from build123d import *

# Parameters (mm, degrees)
F0_W      = 27
F0_H      = 15.9
F0_W_2    = 15.9
F0_H_2    = 27
F0_W_3    = 3
F0_H_3    = 3
F1_DEPTH  = 21.9
F2_DEPTH  = 51.8
F3_R      = 7.95
F6_DEPTH  = 30
F7_DEPTH  = 30
F4_R      = 7.9
F8_DEPTH  = 30
F10_DEPTH = 58.2
F11_W     = 3
F11_H     = 13.3
F13_R     = 1.5
F17_DEPTH = 51.9


with BuildPart() as f1:
    # F0 (on Front) → F1 (new body)
    with BuildSketch(Plane.XZ):
        with BuildLine():
            Line((-34.3576915575, 15.9), (-42.3076915575, 15.9))
            Line((-42.3076915575, 15.9), (-42.3076915575, 7.9499999931))
            ThreePointArc((-42.3076915575, 7.9499999931), (-39.9791904704, 13.571498908), (-34.3576915575, 15.9))
        make_face()
        with BuildLine():
            ThreePointArc((-34.3576915575, 15.9), (-39.9791904704, 13.571498908), (-42.3076915575, 7.9499999931))
            ThreePointArc((-42.3076915575, 7.9499999931), (-39.9791904655, 2.3285010871), (-34.3576915575, 0))
            ThreePointArc((-34.3576915575, 0), (-28.7361926471, 2.3285010896), (-26.4076915575, 7.95))
            ThreePointArc((-26.4076915575, 7.95), (-28.7361926471, 13.5714989104), (-34.3576915575, 15.9))
        make_face()
        Polygon((-42.3076915575, 18.9), (-42.3076915575, 45.9), (-26.4076915575, 45.9), (-26.4076915575, 18.9), (-23.4076915575, 18.9), (-23.4076915575, 48.9), (-45.3076915575, 48.9), (-45.3076915575, 18.9), align=None)
        with Locations((-9.9076915575, 7.95)):
            Rectangle(F0_W, F0_H)
        with Locations((-34.3576915575, 32.4)):
            Rectangle(F0_W_2, F0_H_2)
        with BuildLine():
            ThreePointArc((-34.3576915575, 0), (-39.9791904655, 2.3285010871), (-42.3076915575, 7.9499999931))
            Line((-42.3076915575, 7.9499999931), (-42.3076915575, 0))
            Line((-42.3076915575, 0), (-34.3576915575, 0))
        make_face()
        with BuildLine():
            Line((-26.4076915575, 0), (-26.4076915575, 7.95))
            ThreePointArc((-26.4076915575, 7.95), (-28.7361926471, 2.3285010896), (-34.3576915575, 0))
            Line((-34.3576915575, 0), (-26.4076915575, 0))
        make_face()
        with BuildLine():
            Line((-26.4076915575, 7.95), (-26.4076915575, 15.9))
            Line((-26.4076915575, 15.9), (-34.3576915575, 15.9))
            ThreePointArc((-34.3576915575, 15.9), (-28.7361926471, 13.5714989104), (-26.4076915575, 7.95))
        make_face()
        Polygon((6.5923084425, 18.9), (-23.4076915575, 18.9), (-23.4076915575, 15.9), (3.5923084425, 15.9), (3.5923084425, 0), (-23.4076915575, 0), (-23.4076915575, -3), (6.5923084425, -3), align=None)
        Polygon((-26.4076915575, 18.9), (-42.3076915575, 18.9), (-42.3076915575, 15.9), (-34.3576915575, 15.9), (-26.4076915575, 15.9), align=None)
        Polygon((-23.4076915575, 15.9), (-26.4076915575, 15.9), (-26.4076915575, 7.95), (-26.4076915575, 0), (-23.4076915575, 0), align=None)
        Polygon((-42.3076915575, 15.9), (-42.3076915575, 18.9), (-45.3076915575, 18.9), (-45.3076915575, -3), (-23.4076915575, -3), (-23.4076915575, 0), (-26.4076915575, 0), (-34.3576915575, 0), (-42.3076915575, 0), (-42.3076915575, 7.9499999931), align=None)
        with Locations((-24.9076915575, 17.4)):
            Rectangle(F0_W_3, F0_H_3)
    extrude(amount=F1_DEPTH)

    # F0 (on Front) → F2 (join)
    with BuildSketch(Plane.XZ):
        Polygon((-42.3076915575, 15.9), (-42.3076915575, 18.9), (-45.3076915575, 18.9), (-45.3076915575, -3), (-23.4076915575, -3), (-23.4076915575, 0), (-26.4076915575, 0), (-34.3576915575, 0), (-42.3076915575, 0), (-42.3076915575, 7.9499999931), align=None)
        with BuildLine():
            ThreePointArc((-34.3576915575, 15.9), (-39.9791904704, 13.571498908), (-42.3076915575, 7.9499999931))
            ThreePointArc((-42.3076915575, 7.9499999931), (-39.9791904655, 2.3285010871), (-34.3576915575, 0))
            ThreePointArc((-34.3576915575, 0), (-28.7361926471, 2.3285010896), (-26.4076915575, 7.95))
            ThreePointArc((-26.4076915575, 7.95), (-28.7361926471, 13.5714989104), (-34.3576915575, 15.9))
        make_face()
        Polygon((-26.4076915575, 18.9), (-42.3076915575, 18.9), (-42.3076915575, 15.9), (-34.3576915575, 15.9), (-26.4076915575, 15.9), align=None)
        Polygon((-23.4076915575, 15.9), (-26.4076915575, 15.9), (-26.4076915575, 7.95), (-26.4076915575, 0), (-23.4076915575, 0), align=None)
        with Locations((-24.9076915575, 17.4)):
            Rectangle(F0_W_3, F0_H_3)
        with BuildLine():
            Line((-26.4076915575, 7.95), (-26.4076915575, 15.9))
            Line((-26.4076915575, 15.9), (-34.3576915575, 15.9))
            ThreePointArc((-34.3576915575, 15.9), (-28.7361926471, 13.5714989104), (-26.4076915575, 7.95))
        make_face()
        with BuildLine():
            Line((-34.3576915575, 15.9), (-42.3076915575, 15.9))
            Line((-42.3076915575, 15.9), (-42.3076915575, 7.9499999931))
            ThreePointArc((-42.3076915575, 7.9499999931), (-39.9791904704, 13.571498908), (-34.3576915575, 15.9))
        make_face()
        with BuildLine():
            ThreePointArc((-34.3576915575, 0), (-39.9791904655, 2.3285010871), (-42.3076915575, 7.9499999931))
            Line((-42.3076915575, 7.9499999931), (-42.3076915575, 0))
            Line((-42.3076915575, 0), (-34.3576915575, 0))
        make_face()
        with BuildLine():
            Line((-26.4076915575, 0), (-26.4076915575, 7.95))
            ThreePointArc((-26.4076915575, 7.95), (-28.7361926471, 2.3285010896), (-34.3576915575, 0))
            Line((-34.3576915575, 0), (-26.4076915575, 0))
        make_face()
    extrude(amount=F2_DEPTH)

    # F3 (on face) → F6 (cut)
    with BuildSketch(Plane.XZ.offset(51.8)):
        with Locations((-34.3576915575, 7.95)):
            Circle(F3_R)
    extrude(amount=-F6_DEPTH, mode=Mode.SUBTRACT)

    # F5 (on face) → F7 (cut)
    with BuildSketch(Plane.YZ.offset(6.5923084425)):
        with BuildLine():
            ThreePointArc((-3, 7.95), (-5.3285010896, 13.5714989104), (-10.95, 15.9))
            ThreePointArc((-10.95, 15.9), (-16.5714989104, 13.5714989104), (-18.9, 7.95))
            ThreePointArc((-18.9, 7.95), (-16.5714989104, 2.3285010896), (-10.95, 0))
            ThreePointArc((-10.95, 0), (-5.3285010896, 2.3285010896), (-3, 7.95))
        make_face()
    extrude(amount=-F7_DEPTH, mode=Mode.SUBTRACT)

    # F4 (on face) → F8 (cut)
    with BuildSketch(Plane.XY.offset(48.9)):
        with Locations((-34.3576915575, -10.9)):
            Circle(F4_R)
    extrude(amount=-F8_DEPTH, mode=Mode.SUBTRACT)

    # F9 (on face) → F10 (join)
    with BuildSketch(Plane.XZ.offset(51.8)):
        Polygon((-51.6076915575, -3), (-45.3076915575, -3), (-45.3076915575, 0), (-48.6076915575, 0), (-48.6076915575, 13.3), (-51.6076915575, 13.3), align=None)
    extrude(amount=-F10_DEPTH)

    # F11 (on face) → F12 (join, up to the next surface of F1)
    with BuildSketch(Plane.YZ.offset(6.5923084425)):
        Polygon((6.4, -3), (6.4, 0), (3.4, 0), (0, 0), (0, -3), align=None)
        with Locations((4.9, 6.65)):
            Rectangle(F11_W, F11_H)
    extrude(until=Until.NEXT, dir=(-1, 0, 0))

    # F13
    f13_edges = [f1.edges().sort_by_distance(p)[0] for p in [
        (6.592308, 3.4, 6.65),
        (-48.607692, -51.8, 6.65),
    ]]
    fillet(f13_edges, radius=F13_R)


with BuildPart() as f14_1:
    # F14: instance of F1
    add(f1.part.mirror(Plane(origin=(6.5923084425, -9.0672909783, 7.3023649608), x_dir=(0, 1, 0), z_dir=(1, 0, 0))))

    # F16 (on face) → F17 (join)
    with BuildSketch(Plane.XZ.offset(51.8)):
        Polygon((64.7923084425, -9.3), (64.7923084425, -3), (61.7923084425, -3), (61.7923084425, -6.3), (48.4923084425, -6.3), (48.4923084425, -9.3), align=None)
    extrude(amount=-F17_DEPTH)


solid = f14_1.part
Here's how the part is built. I have some questions about the finished solid (model axes, mm). A direction names the side the tool comes from. Give positions to 0.01 mm unless a question says otherwise; leave off trailing zeros. Loops run counter-clockwise (first coordinate to the right, second up) from the corner with the lowest first, then second, coordinate; pieces in that order, holes last. Notation, with made-up numbers: (41, -0.75) -> (68, -0.75) arc R27 cw to (68, 24.25) -> close; hole circle Ø5 at (22.25, 0.5). An arc over 180 degrees is marked (long way). One line per item, written item: value.
Q1. Suppose I cut it at A-A on y = -45.5. Please give me the cut outline in (x, z).
Answers follow:
outline: (36.59, -3) -> (61.79, -3) -> (61.79, -6.3) -> (48.49, -6.3) -> (48.49, -9.3) -> (64.79, -9.3) -> (64.79, 13.3) -> (61.79, 13.3) -> (61.79, 0) -> (58.49, 0) -> (58.49, 18.9) -> (36.59, 18.9) -> close; hole circle Ø15.9 at (47.54, 7.95)
Q2. Suppose I cut it at B-B on x = 29. Please give me the cut outline in (y, z), then the cut area to 3 significant figures.
Answers follow:
outline: (-21.9, -3) -> (6.4, -3) -> (6.4, 13.3) -> (3.4, 13.3) -> (3.4, 0) -> (0, 0) -> (0, 18.9) -> (-21.9, 18.9) -> close; hole circle Ø15.9 at (-10.95, 7.95)
area: 340 mm^2
Q3. I'm going to push flat-ended pins straight in: pin 1 Ø17.5 at (x, y) = (31.5, -33) entering from -Z; pin 2 Ø5 at (y, z) = (-33.5, 16.5) entering from -X; pin 3 Ø11 at (x, z) = (50.5, 35) entering from -Y; pin 4 Ø10 at (x, z) = (25.5, 26) entering from +Y. Where does each tip first touch, or does it pass through?
Answers follow:
pin 1: z = -3
pin 2: x = 36.59
pin 3: y = -21.9
pin 4: through
Q4. Suppose I cut it at D-D on y = -20.5. Please give me the cut outline in (x, z).
Answers follow:
outline: (6.59, -3) -> (61.79, -3) -> (61.79, -6.3) -> (48.49, -6.3) -> (48.49, -9.3) -> (64.79, -9.3) -> (64.79, 13.3) -> (61.79, 13.3) -> (61.79, 0) -> (58.49, 0) -> (58.49, 48.9) -> (36.59, 48.9) -> (36.59, 18.9) -> (6.59, 18.9) -> close
Q5. If I drill on line 1 along Z through (x, y) = (54, -11.5); line 2 along Y through (x, z) = (18, 12.5); line 3 along Y through (x, z) = (54, 3.5), over which ranges is the centre line in solid material (lowest first)?
Answers follow:
line 1: -9.3 to -6.3, -3 to 18.9
line 2: -21.9 to -17.47, -4.43 to 0, 3.4 to 6.4
line 3: -21.8 to 0, 3.4 to 6.4
Q6. On a 3-axis mill with a long thin cutter (end or side, diameter ignored), from which of +Z, -Z, +X, -X, +Y, -Y can I reach the whole of each face in a straight line? I mean faces 4 (the face through (36.592, -37, 8)), 5 (the face through (58, 0.1, -8)), 6 (the face through (47, 2, 0)), 7 (the face through (55.485, -37.01, 8.3)), 8 (the face through (21, -11, 18.9)). Say none if no direction works.
Answers follow:
face 4: +Z, -Z, -X, -Y
face 5: -Z, +X, -X, +Y
face 6: +Z
face 7: -Y
face 8: +Z, -X, +Y, -Y
Q7. Suppose I cut it at C-C on z = 9. Please give me the cut outline in (x, y), then the cut area to 3 significant figures.
Answers follow:
outline: (6.59, -21.9) -> (36.59, -21.9) -> (36.59, -51.8) -> (39.66, -51.8) -> (39.66, -21.8) -> (55.42, -21.8) -> (55.42, -51.8) -> (58.49, -51.8) -> (58.49, 0) -> (6.59, 0) -> (6.59, -3.07) -> (36.59, -3.07) -> (36.59, -18.83) -> (6.59, -18.83) -> close; (6.59, 4.9) arc R1.5 ccw to (8.09, 3.4) -> (61.79, 3.4) -> (61.79, -50.3) arc R1.5 ccw to (63.29, -51.8) -> (64.79, -51.8) -> (64.79, 6.4) -> (6.59, 6.4) -> close
area: 1,190 mm^2
Q8. We'd pull the mould along Y, two halves only. Please class faces 1 (the face through (36.592, -11, 34)), 2 (the face through (36.592, -11, 8)), 3 (the face through (22, -21.9, 8)): pulls with the +Y half, pulls with the -Y half, needs draft (parallel to the pull), parting line crosses it, or undercut.
Answers follow:
face 1: needs draft
face 2: undercut
face 3: pulls with the -Y half
